Here's how the part is built. I have some questions about the finished solid (model axes, mm). A direction names the side the tool comes from. Coordinates: 2 decimals unless noted, no trailing zeros. Write each loop counter-clockwise with the first axis right and the second up, starting at its lowest first coordinate (ties: lowest second). Pieces come first, ordered by that corner, then holes.
Item 1: If we section it at B-B (y = 2.1): Please give me the cut outline in (x, z), then the cut area to 3 significant figures.
Item 2: If I drill on line 1 (X direction, y = 1.45, z = 0); line 2 (X direction, y = 1.8, z = 21.5); line 3 (X direction, y = 1.8, z = 9), over which ranges is the centre line in solid material (lowest first)?
Item 3: If we section it at A-A (z = 0): Please give me the cut outline in (x, y), then the cut area to 3 significant figures.
Item 4: I'm going to push flat-ended pins straight in: pin 1 Ø1.9 at (x, z) = (37.5, 0) entering from +Y; pin 2 Ø0.5 at (x, y) = (37.5, 1) entering from +Z; pin 3 Ø0.5 at (x, y) = (-37.5, 1.5) entering from -Z. Where does each tip first touch, or does it pass through?
Item 5: For faces 1 (the face through (-34, 1, 22)), 2 (the face through (0, 1, -34)), 3 (the face through (34, 1, 22)), 4 (the face through (-34, 1, -22)), 5 (the face through (34, 1, -22)), which set-ups out of +Z, -Z, +X, -X, +Y, -Y let a thin tool reach every point of the face, with its end or its side?
Item 6: If we section it at C-C (z = -23): Please give me the cut outline in (x, y).
Item 7: We'd pull the mould along Z, two halves only. Please class faces 6 (the face through (36.08, 1.52, 0.74)), 7 (the face through (34.86, 1.48, 10.9)), 8 (the face through (33.14, 1.52, -33.1)): +Z half, -Z half, draft (parallel to the pull), parting line (faces both ways), or undercut.
from build123d import *

# Parameters (mm, degrees)
SKETCH1_W           = 68
SKETCH1_H           = 68
BOSS_EXTRUDE1_DEPTH = 3
SKETCH2_W           = 7
SKETCH2_H           = 20
SKETCH2_R           = 1.6
BOSS_EXTRUDE2_DEPTH = 3
FILLET1_R           = 3


with BuildPart() as part:
    # Sketch1 → Boss-Extrude1 (new body)
    with BuildSketch(Plane(origin=(0, 0, 0), x_dir=(1, 0, 0), z_dir=(0, 1, 0))):
        Rectangle(SKETCH1_W, SKETCH1_H)
    extrude(amount=BOSS_EXTRUDE1_DEPTH)

    # Sketch2 → Boss-Extrude2 (add)
    # profile 1 of 2: a face of its own
    with BuildSketch(Plane(origin=(0, 3, 0), x_dir=(1, 0, 0), z_dir=(0, 1, 0))):
        with Locations((37.5, 0)):
            Rectangle(SKETCH2_W, SKETCH2_H)
        with Locations(Location((37.5, 0, 0), (0, 0, 270))):
            Circle(SKETCH2_R, mode=Mode.SUBTRACT)
    # profile 2 of 2: a face of its own
    with BuildSketch(Plane(origin=(0, 3, 0), x_dir=(1, 0, 0), z_dir=(0, 1, 0))):
        with Locations((-37.5, 0)):
            Rectangle(SKETCH2_W, SKETCH2_H)
        with Locations(Location((-37.5, 0, 0), (0, 0, 270))):
            Circle(SKETCH2_R, mode=Mode.SUBTRACT)
    extrude(amount=-BOSS_EXTRUDE2_DEPTH)

    # Fillet1
    fillet1_edges = [part.edges().sort_by_distance(p)[0] for p in [
        (34, 1.5, 10),
        (41, 1.5, 10),
        (41, 1.5, -10),
        (34, 1.5, -10),
        (-41, 1.5, -10),
        (-41, 1.5, 10),
        (-34, 1.5, 10),
        (-34, 1.5, -10),
        (-34, 1.5, 34),
        (34, 1.5, 34),
        (34, 1.5, -34),
        (-34, 1.5, -34),
    ]]
    fillet(fillet1_edges, radius=FILLET1_R)


solid = part.part
Answer list:
1. outline: (-41, -7) arc R3 ccw to (-38, -10) - (-37, -10) arc R3 cw to (-34, -13) - (-34, -31) arc R3 ccw to (-31, -34) - (31, -34) arc R3 ccw to (34, -31) - (34, -13) arc R3 cw to (37, -10) - (38, -10) arc R3 ccw to (41, -7) - (41, 7) arc R3 ccw to (38, 10) - (37, 10) arc R3 cw to (34, 13) - (34, 31) arc R3 ccw to (31, 34) - (-31, 34) arc R3 ccw to (-34, 31) - (-34, 13) arc R3 cw to (-37, 10) - (-38, 10) arc R3 ccw to (-41, 7) - close; hole circle Ø3.2 at (-37.5, 0); hole circle Ø3.2 at (37.5, 0)
1. area: 4,880 mm2
2. line 1: x = -41 to -39.1, -35.9 to 35.9, 39.1 to 41
2. line 2: x = -34 to 34
2. line 3: x = -40.24 to 40.24
3. outline: (-41, 0) - (-39.1, 0) - (-39.1, 3) - (-41, 3) - close; (-35.9, 0) - (35.9, 0) - (35.9, 3) - (-35.9, 3) - close; (39.1, 0) - (41, 0) - (41, 3) - (39.1, 3) - close
3. area: 227 mm2
4. pin 1: passes through
4. pin 2: stops at z = 10
4. pin 3: stops at z = -10
5. face 1: +Z, -X, +Y, -Y
5. face 2: -Z, +X, -X, +Y, -Y
5. face 3: +Z, +X, +Y, -Y
5. face 4: -Z, -X, +Y, -Y
5. face 5: -Z, +X, +Y, -Y
6. outline: (-34, 0) - (34, 0) - (34, 3) - (-34, 3) - close
7. face 6: undercut
7. face 7: +Z half
7. face 8: -Z half
